Autodesk Inventor part; units mm, degrees
ref_plane "YZ Plane" through (0, 0, 0) normal (1, 0, 0) x (0, 1, 0)
ref_plane "XZ Plane" through (0, 0, 0) normal (0, 1, 0) x (-1, 0, 0)
ref_plane "XY Plane" through (0, 0, 0) normal (0, 0, 1) x (1, 0, 0)
sketch "Sketch1" plane through (0, 0, 0) normal (0, 1, 0) x (-1, 0, 0)
  line L0 (0, 0) -> (40, 0)
  line L1 (40, 0) -> (40, -40)
  line L2 (40, -40) -> (0, -40)
  line L3 (0, -40) -> (0, 0)
  dimension "d0" = 40
extrude "Extrusion1" add sketch "Sketch1" along normal blind 4
sketch "Sketch2" plane through (-40, 0, 0) normal (0, 0, 1) x (1, 0, 0)
  circle A0 centre (2, 1.9356) radius 1.4452
  line L0 (0, 0) -> (0, 4)
  line L1 (0, 4) -> (40, 4)
  line L2 (20, 17.4012) -> (20, -9.9341)
  circle A1 centre (38, 1.9356) radius 1.4452
  point P0 (40, 0)
  dimension "d3" = 2
  dimension "d4" = 40
  dimension "d5" = 20
extrude "Extrusion2" add sketch "Sketch2" along normal blind 2.54
equation "\"d5\" = 0.5 * d4"
properties part number "SP1848-27145 4.8V Seebeck Thermoelectric Power Generator TEG Peltier Module"
Verification items for the finished model (mm, model axes). A direction names the side the tool comes from. Round coordinates to 2 decimals unless told otherwise and drop trailing zeros. Write each loop counter-clockwise with the first axis right and the second up, starting at its lowest first coordinate (ties: lowest second). Pieces come first, ordered by that corner, then holes.
1. Draft check along X on faces 1 (the cylindrical face through (-39.444, 1.872, 1.252)), 2 (the flat face through (-38, 2, 2.54)), 3 (the flat face through (-40, 2, -20)). Enter one of: +X half, -X half, draft (parallel to the pull), parting line (faces both ways), or undercut.
2. Section check B-B on y = 1.45. Enter the section's corners in (x, z).
3. Section check C-C on x = -5.5. Enter the section's corners in (y, z), plus the area to 3 significant figures.
4. Access from +Z, -Z, +X, -X, +Y, -Y to the whole of each face (thin tool, end or side, straight path). Record for faces 4 (the cylindrical face through (-0.665, 2.489, 1.252)), 5 (the flat face through (-2, 2, 2.54)).
5. Section check A-A on x = -38. Enter the section's corners in (y, z).
6. Gauge pin test, flat end, axial feed: P1, Ø2, axis at x = -22, y = 2.5, coming from the +Z side. Record the tip position at first contact, or that the pin passes through.
7. Scan line: L1, parallel to Z at x = -24, y = 1.95. Record every from-to range of solid material in increasing order.
Answer:
1. face 1: undercut
1. face 2: draft
1. face 3: -X half
2. outline: (-40, -40) - (0, -40) - (0, 0) - (-0.64, 0) - (-0.64, 2.54) - (-3.36, 2.54) - (-3.36, 0) - (-36.64, 0) - (-36.64, 2.54) - (-39.36, 2.54) - (-39.36, 0) - (-40, 0) - close
3. outline: (0, -40) - (4, -40) - (4, 0) - (0, 0) - close
3. area: 160 mm2
4. face 4: +Z
4. face 5: +Z, +X, -X, +Y, -Y
5. outline: (0, -40) - (4, -40) - (4, 0) - (3.38, 0) - (3.38, 2.54) - (0.49, 2.54) - (0.49, 0) - (0, 0) - close
6. P1: stops at z = 0
7. L1: z = -40 to 0
